Check sheet for the modelled part. Datum: model origin and axes. Units: mm. A direction names the side the tool comes from. Give positions to 0.01 mm unless a question says otherwise; leave off trailing zeros. Write each loop counter-clockwise with the first axis right and the second up, starting at its lowest first coordinate (ties: lowest second). Pieces come first, ordered by that corner, then holes. Notation, with made-up numbers: (72, 81.25) -> (82, 81.25) arc R17 cw to (82, 93.25) -> close; hole circle Ø5 at (28.5, 34.25). An arc over 180 degrees is marked (long way). Answer as a JSON object with one key per item and string values.
Autodesk Inventor part; units mm, degrees
ref_plane "YZ Plane" through (0, 0, 0) normal (1, 0, 0) x (0, 1, 0)
ref_plane "XZ Plane" through (0, 0, 0) normal (0, 1, 0) x (-1, 0, 0)
ref_plane "XY Plane" through (0, 0, 0) normal (0, 0, 1) x (1, 0, 0)
sketch "Sketch1" plane through (0, 0, 0) normal (0, 0, 1) x (1, 0, 0)
  line L0 (0, 0) -> (25.4, 0)
  line L1 (25.4, 0) -> (25.4, -25.4)
  line L2 (25.4, -25.4) -> (0, -25.4)
  line L3 (0, -25.4) -> (0, 0)
  line L4 (3.175, -3.175) -> (22.225, -3.175)
  line L5 (22.225, -3.175) -> (22.225, -22.225)
  line L6 (22.225, -22.225) -> (3.175, -22.225)
  line L7 (3.175, -22.225) -> (3.175, -3.175)
  dimension "d0" = 25.4
  dimension "d1" = 25.4
  dimension "d2" = 19.05
  dimension "d3" = 19.05
  dimension "d4" = 3.175
  dimension "d5" = 3.175
extrude "Extrusion1" add sketch "Sketch1" along normal blind 101.6
sketch "Sketch2" plane through (0, -25.4, 0) normal (-1, 0, 0) x (0, 0, 1)
  line L0 (101.6, 25.4) -> (101.6, 0)
  line L1 (101.6, 0) -> (76.2, 25.4)
  line L2 (0, 25.4) -> (101.6, 25.4)
  line L3 (101.6, 0) -> (137.521, 0) construction
  line L4 (76.2, 25.4) -> (101.6, 25.4)
  line L5 (101.6, 25.4) -> (101.6, 0)
  dimension "d8" = 135
extrude "Extrusion2" cut sketch "Sketch2" against normal blind 76.2
properties part number "1x1 mechanical stop" material "Aluminum 6061"
1. Scan lines: L1, parallel to X at y = -4.5, z = 40 (3 decimals); L2, parallel to Y at x = 6.75, z = 8.5 (3 decimals); L3, parallel to Y at x = 18.5, z = 89 (3 decimals). Record each from-to range of solid material in increasing order. Write a range as [from, to].
Determined:
{"L1": "[0, 3.175], [22.225, 25.4]", "L2": "[-25.4, -22.225], [-3.175, 0]", "L3": "[-25.4, -22.225]"}
2. Access from +Z, -Z, +X, -X, +Y, -Y to the whole of each face (thin tool, end or side, straight path). Record for faces 1 (the face through (13, -25.4, 50)), 2 (the face through (13, -22.225, 49)).
Determined:
{"face 1": "+Z, -Z, +X, -X, -Y", "face 2": "+Z, -Z"}
3. Sectioned sample at B-B, the plane x = 11. Enter the section's corners in (y, z) (3 decimals), plus the area to 3 significant figures.
Determined:
{"outline": "(-25.4, 0) -> (-22.225, 0) -> (-22.225, 98.425) -> (-25.4, 101.6) -> close; (-3.175, 0) -> (0, 0) -> (0, 76.2) -> (-3.175, 79.375) -> close", "area": "565 mm^2"}
4. Sectioned sample at C-C, the plane z = 54.5. Enter the section's corners in (x, y) (3 decimals), plus the area to 3 significant figures.
Determined:
{"outline": "(0, -25.4) -> (25.4, -25.4) -> (25.4, 0) -> (0, 0) -> close; hole (3.175, -22.225) -> (22.225, -22.225) -> (22.225, -3.175) -> (3.175, -3.175) -> close", "area": "282 mm^2"}
5. Mould release check, pull along X, two halves, no side actions. Record for faces 3 (the face through (13, 0, 38)), 4 (the face through (3.175, -13, 49)), 5 (the face through (25.4, -13, 39)), 6 (the face through (13, -3.175, 39)): released by +X, released by -X, zero draft, split by the parting line, or undercut.
Determined:
{"face 3": "zero draft", "face 4": "undercut", "face 5": "released by +X", "face 6": "undercut"}
6. Sectioned sample at A-A, the plane y = -9.25. Enter the section's corners in (x, z) (3 decimals), plus the area to 3 significant figures.
Determined:
{"outline": "(0, 0) -> (3.175, 0) -> (3.175, 85.45) -> (0, 85.45) -> close; (22.225, 0) -> (25.4, 0) -> (25.4, 85.45) -> (22.225, 85.45) -> close", "area": "543 mm^2"}
7. Go/stop test with flat-tipped pins: P1, Ø2, axis at y = -14, z = 68, coming from the -X side; P2, Ø6, axis at x = 20, y = -5.5, coming from the +Z side. Record where each tip stops, or that it passes through.
Determined:
{"P1": "x = 0", "P2": "z = 83.71"}
